from build123d import *

# Parameters (mm, degrees)
EXTRUDE_THIN1_DEPTH = 9.75
CUT_EXTRUDE1_DEPTH  = 2
FILLET2_R           = 2


with BuildPart() as part:
    # Sketch1 → Extrude-Thin1 (new, symmetric)
    with BuildSketch(Plane(origin=(0, 0, 0), x_dir=(0, 0, -1), z_dir=(1, 0, 0))):
        with BuildLine():
            Line((0, 0), (13.5, 0))
            ThreePointArc((13.5, 0), (14.560660172, 0.439339828), (15, 1.5))
            Line((15, 1.5), (15, 16.5))
            ThreePointArc((15, 16.5), (16.025126266, 18.974873734), (18.5, 20))
            Line((18.5, 20), (32, 20))
            Line((32, 20), (32, 18))
            Line((32, 18), (18.5, 18))
            ThreePointArc((18.5, 18), (17.439339828, 17.560660172), (17, 16.5))
            Line((17, 16.5), (17, 1.5))
            ThreePointArc((17, 1.5), (15.974873734, -0.974873734), (13.5, -2))
            Line((13.5, -2), (0, -2))
            Line((0, -2), (0, 0))
        make_face()
    extrude(amount=EXTRUDE_THIN1_DEPTH, both=True)

    # Sketch2 → Cut-Extrude1 (cut)
    with BuildSketch(Plane(origin=(0, 20, 0), x_dir=(1, 0, 0), z_dir=(0, 1, 0))):
        with BuildLine():
            Line((-2.9, 29.45), (2.9, 29.45))
            Line((2.9, 29.45), (2.9, 27.15))
            ThreePointArc((2.9, 27.15), (2.973223305, 26.973223305), (3.15, 26.9))
            Line((3.15, 26.9), (5.3, 26.9))
            Line((5.3, 26.9), (5.3, 21.4))
            Line((5.3, 21.4), (3.15, 21.4))
            ThreePointArc((3.15, 21.4), (2.973223305, 21.326776695), (2.9, 21.15))
            Line((2.9, 21.15), (2.9, 18.85))
            Line((2.9, 18.85), (-2.9, 18.85))
            Line((-2.9, 18.85), (-2.9, 21.15))
            ThreePointArc((-2.9, 21.15), (-2.973223305, 21.326776695), (-3.15, 21.4))
            Line((-3.15, 21.4), (-5.3, 21.4))
            Line((-5.3, 21.4), (-5.3, 26.9))
            Line((-5.3, 26.9), (-3.15, 26.9))
            ThreePointArc((-3.15, 26.9), (-2.973223305, 26.973223305), (-2.9, 27.15))
            Line((-2.9, 27.15), (-2.9, 29.45))
        make_face()
    extrude(amount=-CUT_EXTRUDE1_DEPTH, mode=Mode.SUBTRACT)

    # Fillet2
    fillet2_edges = [part.edges().sort_by_distance(p)[0] for p in [
        (-9.75, -1, 0),
        (-9.75, 19, -32),
        (9.75, -1, 0),
        (9.75, 19, -32),
    ]]
    fillet(fillet2_edges, radius=FILLET2_R)


solid = part.part
Here's how the part is built. I have some questions about the finished solid (model axes, mm). A direction names the side the tool comes from. Coordinates: 2 decimals unless noted, no trailing zeros. Write each loop counter-clockwise with the first axis right and the second up, starting at its lowest first coordinate (ties: lowest second). Pieces come first, ordered by that corner, then holes.
1) Thinking about a two-plate mould opening in X: for faces 1 (the face through (9.18, 18.99, -31.4)), 2 (the face through (4, 19, -26.9)), 3 (the face through (0, -1, 0)), which applies, +X half, -X half, draft (parallel to the pull), parting line (faces both ways), or undercut?
Filled in:
face 1: +X half
face 2: undercut
face 3: draft
2) Which directions (+Z, -Z, +X, -X, +Y, -Y) give clear straight access to the entire face, cutting with the end or side of a thin tool? Please do faces 4 (the face through (0, 0, -7)), 5 (the face through (0, 18, -30)), 6 (the face through (-2.9, 19, -28)), 7 (the face through (9.15, -0.99, -0.57)).
Filled in:
face 4: +Z, +X, -X, +Y
face 5: -Z, +X, -X, -Y
face 6: +Y, -Y
face 7: +Z, +X, +Y, -Y
3) If I drill on line 1 (X direction, y = 18.25, z = -28.5); line 2 (Y direction, x = 1.25, z = -2); line 3 (Y direction, x = 3, z = -18.5), over which ranges is the centre line in solid material (lowest first)?
Filled in:
line 1: x = -9.75 to -2.9, 2.9 to 9.75
line 2: y = -2 to 0
line 3: y = 18 to 20
4) I'm going to push flat-ended pins straight in: pin 1 (7.5 mm diameter, centred on x = -1, y = 9.5, fed in from -Z); pin 2 (1.6 mm diameter, centred on x = -4, y = 19, fed in from +Z); pin 3 (4.5 mm diameter, centred on x = 2, y = 8, fed in from +Z). Where does each tip first touch, or does it pass through?
Filled in:
pin 1: stops at z = -17
pin 2: stops at z = -15.44
pin 3: stops at z = -15
5) If we section it at B-B (x = 0.5): List the corners of the cut face in (y, z) for me.
Filled in:
outline: (-2, -13.5) arc R3.5 ccw to (1.5, -17) - (16.5, -17) arc R1.5 cw to (18, -18.5) - (18, -18.85) - (20, -18.85) - (20, -18.5) arc R3.5 ccw to (16.5, -15) - (1.5, -15) arc R1.5 cw to (0, -13.5) - (0, 0) - (-2, 0) - close; (18, -32) - (20, -32) - (20, -29.45) - (18, -29.45) - close
6) If we section it at D-D (y = 9): List the corners of the cut face in (x, z) for me.
Filled in:
outline: (-9.75, -17) - (9.75, -17) - (9.75, -15) - (-9.75, -15) - close
7) If we section it at A-A (z = -24.5): List the corners of the cut face in (x, y) for me, plus the area to 3 significant figures.
Filled in:
outline: (-9.75, 18) - (-5.3, 18) - (-5.3, 20) - (-9.75, 20) - close; (5.3, 18) - (9.75, 18) - (9.75, 20) - (5.3, 20) - close
area: 17.8 mm2
8) If we section it at C-C (x = -6.75): List the corners of the cut face in (y, z) for me.
Filled in:
outline: (-2, -13.5) arc R3.5 ccw to (1.5, -17) - (16.5, -17) arc R1.5 cw to (18, -18.5) - (18, -32) - (20, -32) - (20, -18.5) arc R3.5 ccw to (16.5, -15) - (1.5, -15) arc R1.5 cw to (0, -13.5) - (0, 0) - (-2, 0) - close
